For this review, take the finished solid that the model builds, in its own axes (mm). Face numbers are marked on the shaded views. A direction names the side the tool comes from. Round coordinates to 2 decimals unless told otherwise and drop trailing zeros. Order: outer loops, then holes, each group sorted by start corner. A loop starts at its lowest first (then second) coordinate and runs counter-clockwise, first axis right, second up.
from build123d import *

# Parameters (mm, degrees)
SKETCH1_W           = 200
SKETCH1_H           = 70
BOSS_EXTRUDE1_DEPTH = 50
CUT_EXTRUDE5_DEPTH  = 200
CUT_EXTRUDE6_DEPTH  = 5
CUT_EXTRUDE7_DEPTH  = 40
CUT_EXTRUDE8_DEPTH  = 40
CUT_EXTRUDE9_DEPTH  = 40
SKETCH18_W          = 20
SKETCH18_H          = 10
CUT_EXTRUDE10_DEPTH = 20
SKETCH20_W          = 16.096890916
SKETCH20_H          = 2.175255529
BOSS_EXTRUDE2_DEPTH = 5
SKETCH22_W          = 29.287239855
SKETCH22_H          = 12.500651158
CUT_EXTRUDE11_DEPTH = 20
SKETCH23_W          = 32.71404676
SKETCH23_H          = 15.255254966
SKETCH23_W_2        = 29.287239855
SKETCH23_H_2        = 12.500651158
BOSS_EXTRUDE3_DEPTH = 20
SKETCH25_R          = 2.849998823
BOSS_EXTRUDE4_DEPTH = 12
CUT_EXTRUDE12_DEPTH = 12.2
SKETCH28_W          = 4
SKETCH28_H          = 4
CUT_EXTRUDE13_DEPTH = 20


with BuildPart() as part:
    # Sketch1 → Boss-Extrude1 (new body)
    with BuildSketch(Plane(origin=(0, 0, 0), x_dir=(1, 0, 0), z_dir=(0, 1, 0))):
        Rectangle(SKETCH1_W, SKETCH1_H)
    extrude(amount=BOSS_EXTRUDE1_DEPTH)

    # Sketch13 → Cut-Extrude5 (cut)
    with BuildSketch(Plane.ZY.offset(100)):
        with BuildLine():
            Line((-25.356792072, 50), (-35, 50))
            Line((-35, 50), (-35, 0))
            Line((-35, 0), (-25.356792072, 0))
            ThreePointArc((-25.356792072, 0), (-34.489414432, 25), (-25.356792072, 50))
        make_face()
    cut_extrude5 = extrude(amount=-CUT_EXTRUDE5_DEPTH, mode=Mode.SUBTRACT)

    # Mirror1: Cut-Extrude5 across plane
    add(cut_extrude5.mirror(Plane.XY), mode=Mode.SUBTRACT)

    # Sketch14 → Cut-Extrude6 (cut)
    with BuildSketch(Plane.XZ):
        with BuildLine():
            Line((-50.321008897, 22.5), (-50.321008897, -22.5))
            ThreePointArc((-50.321008897, -22.5), (-27.821008897, 0), (-50.321008897, 22.5))
        make_face()
    extrude(amount=-CUT_EXTRUDE6_DEPTH, mode=Mode.SUBTRACT)

    # Sketch15 → Cut-Extrude7 (cut, symmetric)
    with BuildSketch(Plane.XY):
        with BuildLine():
            Line((-14.177189609, 0), (94.750693697, 0))
            ThreePointArc((94.750693697, 0), (40.286752044, 6.203751873), (-14.177189609, 0))
        make_face()
    extrude(amount=CUT_EXTRUDE7_DEPTH, both=True, mode=Mode.SUBTRACT)

    # Sketch16 → Cut-Extrude8 (cut, symmetric)
    with BuildSketch(Plane.XY):
        with BuildLine():
            ThreePointArc((60.094183349, 50), (-19.72974209, 41.127256564), (-100, 43.823614043))
            Line((-100, 43.823614043), (-100, 50))
            Line((-100, 50), (60.094183349, 50))
        make_face()
        with BuildLine():
            Line((100, 0), (100, 4.500444902))
            ThreePointArc((100, 4.500444902), (98.543565753, 1.456434247), (95.499555098, 0))
            Line((95.499555098, 0), (100, 0))
        make_face()
        with BuildLine():
            ThreePointArc((100, 15.440425267), (89.162561497, 39.162561497), (65.440425267, 50))
            Line((65.440425267, 50), (100, 50))
            Line((100, 50), (100, 15.440425267))
        make_face()
    extrude(amount=CUT_EXTRUDE8_DEPTH, both=True, mode=Mode.SUBTRACT)

    # Sketch17 → Cut-Extrude9 (cut, symmetric)
    with BuildSketch(Plane.XY):
        with BuildLine():
            Line((-90.43469404, 42.891964914), (-105.221514707, 46.920266675))
            Line((-105.221514707, 46.920266675), (-103.893419297, 0))
            Line((-103.893419297, 0), (-84.831583922, 0))
            ThreePointArc((-84.831583922, 0), (-89.878284237, 1.691044202), (-93.746012604, 5.347475777))
            ThreePointArc((-93.746012604, 5.347475777), (-98.150815665, 20.070729134), (-100, 35.327104743))
            ThreePointArc((-100, 35.327104743), (-96.78408086, 41.090574557), (-90.43469404, 42.891964914))
        make_face()
    extrude(amount=CUT_EXTRUDE9_DEPTH, both=True, mode=Mode.SUBTRACT)

    # Sketch18 → Cut-Extrude10 (cut)
    with BuildSketch(Plane(origin=(110, 0, 0), x_dir=(0, 0, -1), z_dir=(1, 0, 0))):
        with Locations((0, 30.440425267)):
            Rectangle(SKETCH18_W, SKETCH18_H)
    extrude(amount=-CUT_EXTRUDE10_DEPTH, mode=Mode.SUBTRACT)

    # Sketch20 → Boss-Extrude2 (add)
    with BuildSketch(Plane(origin=(90, 0, 0), x_dir=(0, 0, -1), z_dir=(1, 0, 0))):
        with Locations((0, 32.828238053)):
            Rectangle(SKETCH20_W, SKETCH20_H)
    extrude(amount=BOSS_EXTRUDE2_DEPTH)

    # Sketch22 → Cut-Extrude11 (cut)
    with BuildSketch(Plane(origin=(0, 25, 0), x_dir=(1, 0, 0), z_dir=(0, 1, 0))):
        with Locations((-72.127800153, 0)):
            Rectangle(SKETCH22_W, SKETCH22_H)
    extrude(amount=CUT_EXTRUDE11_DEPTH, mode=Mode.SUBTRACT)

    # Sketch23 → Boss-Extrude3 (add)
    with BuildSketch(Plane(origin=(0, 25, 0), x_dir=(1, 0, 0), z_dir=(0, 1, 0))):
        with Locations((-72.128701672, 0.043393869)):
            Rectangle(SKETCH23_W, SKETCH23_H)
        with Locations((-72.127800153, 0)):
            Rectangle(SKETCH23_W_2, SKETCH23_H_2, mode=Mode.SUBTRACT)
    extrude(amount=BOSS_EXTRUDE3_DEPTH)

    # Sketch25 → Boss-Extrude4 (add)
    with BuildSketch(Plane.XY.offset(-6.250325579)):
        with Locations(Location((-72.128701672, 42.150001177, 0), (0, 0, 90))):
            Circle(SKETCH25_R)
    extrude(amount=BOSS_EXTRUDE4_DEPTH)

    # Sketch27 → Cut-Extrude12 (cut)
    with BuildSketch(Plane(origin=(-105, 0, 0), x_dir=(0, 0, -1), z_dir=(1, 0, 0))):
        with BuildLine():
            Line((-11.180339887, 29.915784745), (11.180339887, 29.915784745))
            ThreePointArc((11.180339887, 29.915784745), (15, 19.915784745), (11.180339887, 9.915784745))
            Line((11.180339887, 9.915784745), (-11.180339887, 9.915784745))
            ThreePointArc((-11.180339887, 9.915784745), (-15, 19.915784745), (-11.180339887, 29.915784745))
        make_face()
    extrude(amount=CUT_EXTRUDE12_DEPTH, mode=Mode.SUBTRACT)

    # Sketch28 → Cut-Extrude13 (cut)
    with BuildSketch(Plane.ZY.offset(92.8)):
        with Locations((-9.180339887, 19.915784745)):
            Rectangle(SKETCH28_W, SKETCH28_H)
        with Locations((9.180339887, 19.915784745)):
            Rectangle(SKETCH28_W, SKETCH28_H)
    extrude(amount=-CUT_EXTRUDE13_DEPTH, mode=Mode.SUBTRACT)


solid = part.part
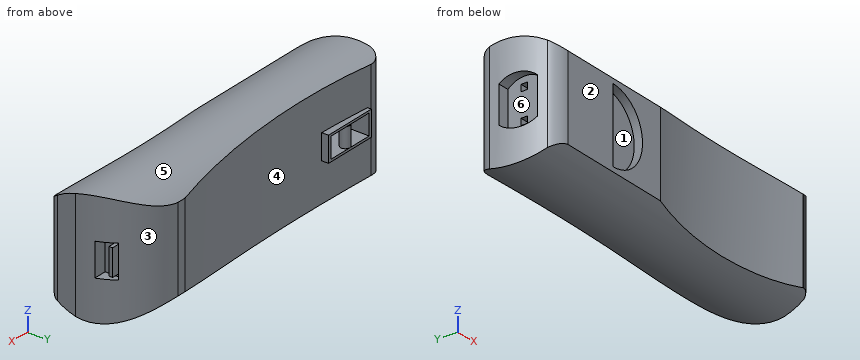
(1) Tool access review of the marked faces 5 and 6: name each direction out of +Z, -Z, +X, -X, +Y, -Y from which nothing blocks a thin tool from reaching the whole face with its end or side.
(2) Add section B-B on y = 8. Give the boundary of the cut face in (x, z), plus the area to 3 significant figures.
(3) Add section A-A on x = -83. Give the boundary of the cut face in (y, z), plus the area to 3 significant figures.
(4) Add section C-C on x = 6. Give the boundary of the cut face in (y, z), plus the area to 3 significant figures.
(5) Wall thickness on L1, parallel to Z at x = -74, y = 43; L2, parallel to Y at x = -44.5, z = -14; L3, parallel to X at y = 38, z = 0: over which ranges is each line inside the solid? List them lowest first.
(6) Clearance check with flat-ended pins moving along their axes: P1, Ø3, axis at x = -55, z = 11, coming from the +Y side; P2, Ø1.1, axis at y = 32.5, z = 0, coming from the +X side; P3, Ø1.2, axis at x = -78.5, z = -8.5, coming from the -Y side; P4, Ø2.5, axis at x = 94, z = -3, coming from the +Y side. State where each tip first meets the part, or that it passes through.
(7) Draft analysis for pull direction X (two halves, no side actions). For the marked faces 1, 2, 3 and 4, state which applies: pulls with the +X half, pulls with the -X half, needs draft (parallel to the pull), parting line crosses it, or undercut.
Here are the results:
1. face 5: +Z, +X, -X
1. face 6: -X
2. outline: (-94.74, -30.57) - (100, -30.57) - (100, 30.57) - (-94.74, 30.57) - close
2. area: 11,900 mm2
3. outline: (0, -25.36) arc R38.78 ccw to (42.28, -30.43) - (42.28, -7.67) - (45, -7.67) - (45, -6.25) - (25, -6.25) - (25, 6.25) - (45, 6.25) - (45, 7.58) - (42.28, 7.58) - (42.28, 30.43) arc R38.78 ccw to (0, 25.36) - close; hole (17.92, -11.18) - (21.92, -11.18) - (21.92, -7.18) - (17.92, -7.18) - close; hole (17.92, 7.18) - (21.92, 7.18) - (21.92, 11.18) - (17.92, 11.18) - close
3. area: 2,490 mm2
4. outline: (3.76, -28.16) arc R38.78 ccw to (42.72, -30.21) - (42.72, 30.21) arc R38.78 ccw to (3.76, 28.16) - close
4. area: 2,550 mm2
5. L1: z = -7.67 to 5.75, 6.25 to 7.58
5. L2: y = 5 to 40.72
5. L3: x = -99.24 to -86.77, -57.48 to 90.28
6. P1: stops at y = 40.92
6. P2: stops at x = 95
6. P3: stops at y = 0
6. P4: stops at y = 33.92
7. face 1: undercut
7. face 2: needs draft
7. face 3: pulls with the +X half
7. face 4: undercut
